Read the model definition and answer for the solid it produces. Units are mm, in the model's axes. Face numbers are marked on the shaded views. Coordinates: 2 decimals unless noted, no trailing zeros. Order: outer loops, then holes, each group sorted by start corner. A loop starts at its lowest first (then second) coordinate and runs counter-clockwise, first axis right, second up. Notation, with made-up numbers: (86, 4.5) -> (98, 4.5) arc R22 cw to (98, 37.5) -> close; hole circle Ø9 at (-12.75, -30.5). An arc over 180 degrees is marked (long way). Answer in a Markdown table with one row per item.
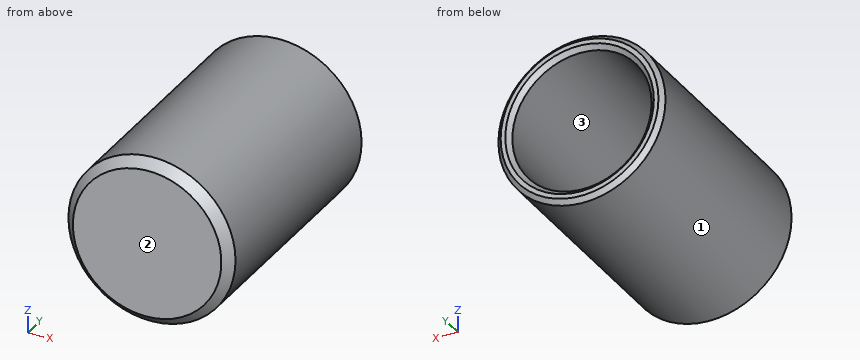
from build123d import *

# Parameters (mm, degrees)
CHAMFER_1_SIZE = 2
CHAMFER_2_SIZE = 1
CHAMFER_3_SIZE = 1


with BuildPart() as part:
    # Эскиз1 → Повернуть1 (revolve)
    with BuildSketch(Plane.XY):
        Polygon((0, 0), (-18, 0), (-18, 55), (-15, 55), (-15, 3), (0, 3), align=None)
    revolve(axis=Axis((0, 3, 0), (0, 1, 0)))

    # Фаска1
    chamfer_1_edges = [part.edges().sort_by_distance(p)[0] for p in [
        (18, 0, 0),
    ]]
    chamfer(chamfer_1_edges, length=CHAMFER_1_SIZE)

    # Фаска2
    chamfer_2_edges = [part.edges().sort_by_distance(p)[0] for p in [
        (15, 55, 0),
        (18, 55, 0),
    ]]
    chamfer(chamfer_2_edges, length=CHAMFER_2_SIZE)

    # Фаска3
    chamfer_3_edges = [part.edges().sort_by_distance(p)[0] for p in [
        (15, 3, 0),
    ]]
    chamfer(chamfer_3_edges, length=CHAMFER_3_SIZE)


solid = part.part
Q1. The part is cut by section B-B (y = 33.5). Write down the section's boundary in (x, z).
Outcome:
| item | result |
|---|---|
| outline | circle Ø36 at (0, 0); hole circle Ø30 at (0, 0) |
Q2. Given pin 1 (10 mm diameter, centred on y = 26, z = 9, fed in from +X); pin 2 (5 mm diameter, centred on x = 0, z = -4, fed in from +Y); pin 3 (4 mm diameter, centred on y = 8, z = -5.5, fed in from -X), each flat-ended and moving along its own axis, determine where each tip first touches the part or whether it passes through.
Outcome:
| item | result |
|---|---|
| pin 1 | x = 17.55 |
| pin 2 | y = 3 |
| pin 3 | x = -17.66 |
Q3. Consider line 1 (Z direction, x = 0, y = 29); line 2 (Z direction, x = 11.5, y = 49.5); line 3 (X direction, y = 18.5, z = 9). Determine where each line is inside the solid, lowest interval first.
Outcome:
| item | result |
|---|---|
| line 1 | -18 to -15, 15 to 18 |
| line 2 | -13.85 to -9.63, 9.63 to 13.85 |
| line 3 | -15.59 to -12, 12 to 15.59 |
Q4. For a pull along Z with two mould halves and no side action, classify the marked faces 1, 2 and 3 as pulls with the +Z half, pulls with the -Z half, needs draft (parallel to the pull), parting line crosses it, or undercut.
Outcome:
| item | result |
|---|---|
| face 1 | parting line crosses it |
| face 2 | needs draft |
| face 3 | undercut |
Q5. The part is cut by section A-A (x = 0). Write down the section's boundary in (y, z), then the cut area to 3 significant figures.
Outcome:
| item | result |
|---|---|
| outline | (0, -16) -> (2, -18) -> (54, -18) -> (55, -17) -> (55, -16) -> (54, -15) -> (4, -15) -> (3, -14) -> (3, 14) -> (4, 15) -> (54, 15) -> (55, 16) -> (55, 17) -> (54, 18) -> (2, 18) -> (0, 16) -> close |
| area | 415 mm² |
Q6. The part is cut by section C-C (z = 0). Write down the section's boundary in (x, y), then the cut area to 3 significant figures.
Outcome:
| item | result |
|---|---|
| outline | (-18, 2) -> (-16, 0) -> (16, 0) -> (18, 2) -> (18, 54) -> (17, 55) -> (16, 55) -> (15, 54) -> (15, 4) -> (14, 3) -> (-14, 3) -> (-15, 4) -> (-15, 54) -> (-16, 55) -> (-17, 55) -> (-18, 54) -> close |
| area | 415 mm² |
